Geometry check sheet. Reference: the model listing, model coordinates, mm. Face numbers are marked on the shaded views. A direction names the side the tool comes from. Coordinates: 2 decimals unless noted, no trailing zeros. Loops run counter-clockwise (first coordinate to the right, second up) from the corner with the lowest first, then second, coordinate; pieces in that order, holes last.
from build123d import *

# Parameters (mm, degrees)
F0_R     = 5
F1_DEPTH = 4
F2_R     = 3
F3_DEPTH = 6
F4_R     = 2
F5_DEPTH = 25
F4_R_2   = 3.5
F6_DEPTH = 2.5
F8_DEPTH = 7


with BuildPart() as f1:
    # F0 (on Front) → F1 (new body)
    with BuildSketch(Plane.XZ):
        Circle(F0_R)
    extrude(amount=F1_DEPTH)

    # F2 (on face) → F3 (join)
    with BuildSketch(Plane.XZ.offset(4)):
        Circle(F2_R)
    extrude(amount=F3_DEPTH)

    # F4 (on face) → F5 (cut)
    with BuildSketch(Plane(origin=(0, 0, 0), x_dir=(-1, 0, 0), z_dir=(0, 1, 0))):
        Circle(F4_R)
    extrude(amount=-F5_DEPTH, mode=Mode.SUBTRACT)

    # F4 (on face) → F6 (cut)
    with BuildSketch(Plane(origin=(0, 0, 0), x_dir=(-1, 0, 0), z_dir=(0, 1, 0))):
        Circle(F4_R_2)
        Circle(F4_R, mode=Mode.SUBTRACT)
    extrude(amount=-F6_DEPTH, mode=Mode.SUBTRACT)

    # F7 (on face) → F8 (join)
    with BuildSketch(Plane.XZ.offset(10)):
        with BuildLine():
            Line((2.49434, 1.666814), (2.49434, 4.33339))
            ThreePointArc((2.49434, 4.33339), (0, 5), (-2.49434, 4.33339))
            Line((-2.49434, 4.33339), (-2.49434, 1.666814))
            ThreePointArc((-2.49434, 1.666814), (0, 3), (2.49434, 1.666814))
        make_face()
    extrude(amount=-F8_DEPTH)


solid = f1.part
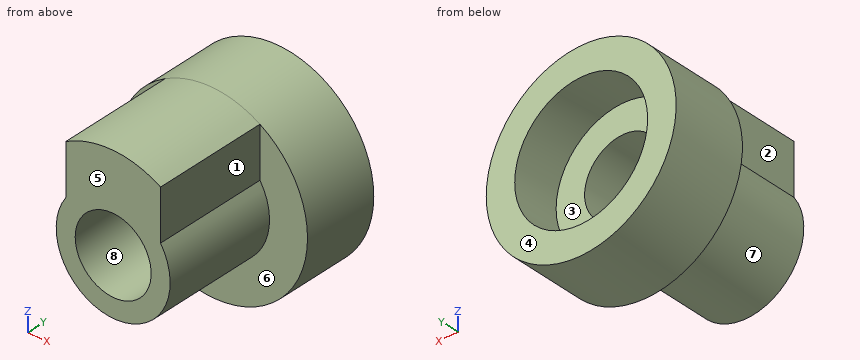
(1) Draft check along Z on the marked faces 6, 7 and 8. Enter one of: +Z half, -Z half, draft (parallel to the pull), parting line (faces both ways), or undercut.
Findings:
face 6: draft
face 7: parting line
face 8: undercut
(2) Sectioned sample at B-B on z = 0. Record the cut outline in (x, y), and give its area (3 significant figures).
Findings:
outline: (-5, -4) - (-3, -4) - (-3, -10) - (-2, -10) - (-2, -2.5) - (-3.5, -2.5) - (-3.5, 0) - (-5, 0) - close; (2, -10) - (3, -10) - (3, -4) - (5, -4) - (5, 0) - (3.5, 0) - (3.5, -2.5) - (2, -2.5) - close
area: 28.5 mm2
(3) Sectioned sample at D-D on x = -1. Record the cut outline in (y, z).
Findings:
outline: (-10, -2.83) - (-4, -2.83) - (-4, -4.9) - (0, -4.9) - (0, -3.35) - (-2.5, -3.35) - (-2.5, -1.73) - (-10, -1.73) - close; (-10, 1.73) - (-2.5, 1.73) - (-2.5, 3.35) - (0, 3.35) - (0, 4.9) - (-10, 4.9) - close
(4) Sectioned sample at C-C on y = -6. Record the cut outline in (x, z).
Findings:
outline: (-2.49, 1.67) arc R3 ccw (long way) to (2.49, 1.67) - (2.49, 4.33) arc R5 ccw to (-2.49, 4.33) - close; hole circle Ø4 at (0, 0)
(5) Access from +Z, -Z, +X, -X, +Y, -Y to the whole of each face (thin tool, end or side, straight path). Record for the marked faces 1, 2, 3, 4 and 5.
Findings:
face 1: +Z, +X, -Y
face 2: +Z, -X, -Y
face 3: +Y
face 4: +Z, -Z, +X, -X, +Y
face 5: +Z, -Z, +X, -X, -Y
(6) Scan lines: L1, parallel to Z at x = 0, y = -1.6; L2, parallel to Z at x = 1.5, y = -8.75; L3, parallel to Y at x = -2.75, z = -1.75. Record each from-to range of solid material in increasing order.
Findings:
L1: z = -5 to -3.5, 3.5 to 5
L2: z = -2.6 to -1.32, 1.32 to 4.77
L3: y = -4 to -2.5
(7) Gauge pin test, flat ends, axial feed: pin 1 Ø3 at (y, z) = (-7.5, 3.5) entering from -X; pin 2 Ø0.8 at (y, z) = (-8, 3) entering from +X; pin 3 Ø1.5 at (y, z) = (-5.5, -2.5) entering from -X. Record the tip position at first contact, or that the pin passes through.
Findings:
pin 1: stops at x = -2.49
pin 2: stops at x = 2.49
pin 3: stops at x = -2.44
(8) Sectioned sample at A-A on x = 0. Record the cut outline in (y, z), and give its area (3 significant figures).
Findings:
outline: (-10, -3) - (-4, -3) - (-4, -5) - (0, -5) - (0, -3.5) - (-2.5, -3.5) - (-2.5, -2) - (-10, -2) - close; (-10, 2) - (-2.5, 2) - (-2.5, 3.5) - (0, 3.5) - (0, 5) - (-10, 5) - close
area: 40.5 mm2
